Answer from the drawing. Dimensions are ordinates in mm from the lowest x, y and z of the part. A direction names the side the tool comes from. Coordinates: 2 decimals unless noted, no trailing zeros. Write each loop counter-clockwise with the first axis right and the second up, starting at its lowest first coordinate (ties: lowest second). Pieces come first, ordered by that corner, then holes.
(1) Find the intervals of material crossed by probe 1 along Z at (x, y) = (34.25, 32); probe 2 along Y at (x, z) = (32.9, 11.5); probe 3 along Z at (x, y) = (11.5, 21.5), in increasing order.
(2) Section A-A on z = 11.5 is taken. Write down the section's boundary in (x, y), then the cut area to 3 significant figures.
(3) Section D-D on y = 32 is taken. Write down the section's boundary in (x, z).
(4) Section C-C on y = 25 is taken. Write down the section's boundary in (x, z).
(5) Section B-B on x = 25 is taken. Write down the section's boundary in (y, z), then the cut area to 3 significant figures.
(6) Given pin 1 (6 mm diameter, centred on x = 23, y = 10.5, fed in from -Z); pin 2 (3 mm diameter, centred on y = 18, z = 32.5, fed in from -X); pin 3 (8 mm diameter, centred on y = 22, z = 10, fed in from +X); pin 4 (1 mm diameter, centred on x = 33, z = 7, fed in from +Y), each flat-ended and moving along its own axis, determine where each tip first touches the part or whether it passes through.
(7) Which of the six approach directions +Z, -Z, +X, -X, +Y, -Y give full straight-line access (tool end or side, diameter ignored) to the marked faces 1, 2, 3 and 4?
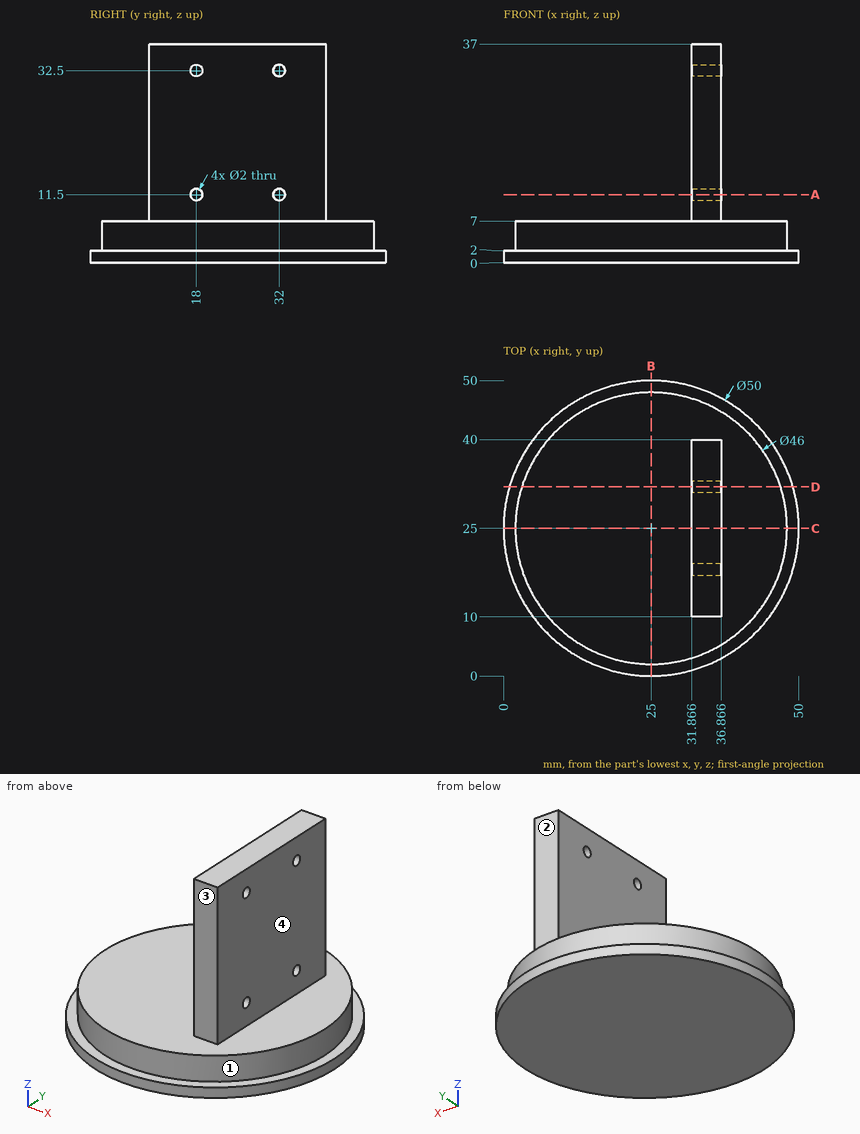
Response:
1. probe 1: z = 0 to 10.5, 12.5 to 31.5, 33.5 to 37
1. probe 2: y = 10 to 17, 19 to 31, 33 to 40
1. probe 3: z = 0 to 7
2. outline: (31.87, 10) - (36.87, 10) - (36.87, 17) - (31.87, 17) - close; (31.87, 19) - (36.87, 19) - (36.87, 31) - (31.87, 31) - close; (31.87, 33) - (36.87, 33) - (36.87, 40) - (31.87, 40) - close
2. area: 130 mm2
3. outline: (1, 0) - (49, 0) - (49, 2) - (46.91, 2) - (46.91, 7) - (36.87, 7) - (36.87, 10.5) - (31.87, 10.5) - (31.87, 7) - (3.09, 7) - (3.09, 2) - (1, 2) - close; (31.87, 12.5) - (36.87, 12.5) - (36.87, 31.5) - (31.87, 31.5) - close; (31.87, 33.5) - (36.87, 33.5) - (36.87, 37) - (31.87, 37) - close
4. outline: (0, 0) - (50, 0) - (50, 2) - (48, 2) - (48, 7) - (36.87, 7) - (36.87, 37) - (31.87, 37) - (31.87, 7) - (2, 7) - (2, 2) - (0, 2) - close
5. outline: (0, 0) - (50, 0) - (50, 2) - (48, 2) - (48, 7) - (2, 7) - (2, 2) - (0, 2) - close
5. area: 330 mm2
6. pin 1: stops at z = 0
6. pin 2: stops at x = 31.87
6. pin 3: stops at x = 48
6. pin 4: stops at y = 46.74
7. face 1: +Z
7. face 2: +Z, +X, -X, +Y
7. face 3: +Z, +X, -X, -Y
7. face 4: +Z, +X, +Y, -Y
